from build123d import *

# Parameters (mm, degrees)
CHAMFER_1_SIZE = 0.1


with BuildPart() as part:
    # 草图1 → 旋转1 (revolve)
    with BuildSketch(Plane.XY, mode=Mode.PRIVATE) as revolve_1_sk:
        Polygon((0, 1.5), (0, 2), (-0.2, 2), (-0.2, 3.5), (0, 3.5), (0, 4), (-4, 4), (-4, 3.5), (-3.8, 3.5), (-3.8, 2), (-4, 2), (-4, 1.5), align=None)
    revolve(revolve_1_sk.sketch.rotate(Axis((-16.444867367, 0, 0), (1, 0, 0)), 90), axis=Axis((-16.444867367, 0, 0), (1, 0, 0)))

    # 倒角1
    chamfer_1_edges = [part.edges().sort_by_distance(p)[0] for p in [
        (-4, 0, -4),
        (0, 0, -4),
        (0, 0, -1.5),
        (-4, 0, -1.5),
    ]]
    chamfer(chamfer_1_edges, length=CHAMFER_1_SIZE)


solid = part.part
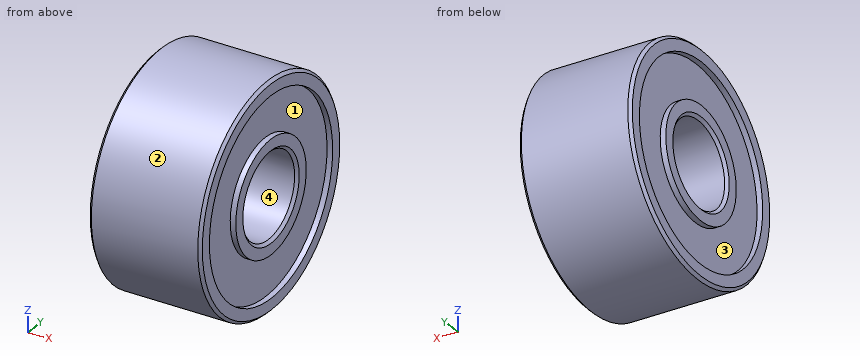
Verification items for the finished model (mm, model axes). Face numbers are marked on the shaded views. A direction names the side the tool comes from. Round coordinates to 2 decimals unless told otherwise and drop trailing zeros. Loops run counter-clockwise (first coordinate to the right, second up) from the corner with the lowest first, then second, coordinate; pieces in that order, holes last. Notation, with made-up numbers: (29, 45.25) - (82, 45.25) arc R26 cw to (82, 60.25) - close; hole circle Ø3 at (73, 15.5). An arc over 180 degrees is marked (long way). Use a Markdown table: item, result. Add a question column.
1. Thickness scan on probe 1 along Y at (x, z) = (-2.6, 0); probe 2 along Y at (x, z) = (-0.15, 0.25); probe 3 along X at (y, z) = (-3, -1.75). Record the ranges inside material, lowest first. Write a range as [from, to].
2. Gauge pin test, flat end, axial feed: pin 1 (1 mm diameter, centred on x = -0.5, z = 1, fed in from +Y). Record the tip position at first contact, or that the pin passes through.
3. Release check for a two-part mould opening along Z. For the marked faces 1 and 2 record: released by +Z, released by -Z, zero draft, split by the parting line, or undercut.
4. Access from +Z, -Z, +X, -X, +Y, -Y to the whole of each face (thin tool, end or side, straight path). Record for the marked faces 3 and 4.
5. Section check C-C, the plane x = -3.05. Record the boundary of the cut face in (y, z), plus the area to 3 significant figures.
Checks:
| question | item | result |
|---|---|---|
| 1 | probe 1 | y = [-4, -1.5], [1.5, 4] |
| 1 | probe 2 | y = [-3.99, -3.49], [-1.98, -1.48], [1.48, 1.98], [3.49, 3.99] |
| 1 | probe 3 | x = [-3.8, -0.2] |
| 2 | pin 1 | stops at y = 3.97 |
| 3 | face 1 | undercut |
| 3 | face 2 | split by the parting line |
| 4 | face 3 | -X |
| 4 | face 4 | +X, -X |
| 5 | outline | circle Ø8 at (0, 0); hole circle Ø3 at (0, 0) |
| 5 | area | 43.2 mm^2 |
